Model file for the job. Use its own axes, mm. Give positions to 0.01 mm unless a question says otherwise; leave off trailing zeros. Loops run counter-clockwise (first coordinate to the right, second up) from the corner with the lowest first, then second, coordinate; pieces in that order, holes last. Notation, with made-up numbers: M 70.25,83.5 L 119.25,83.5 A18 ccw 119.25,109.5 Z; hole C -11,73.25 d1. An arc over 180 degrees is marked long. Answer in a Markdown table with one row per item.
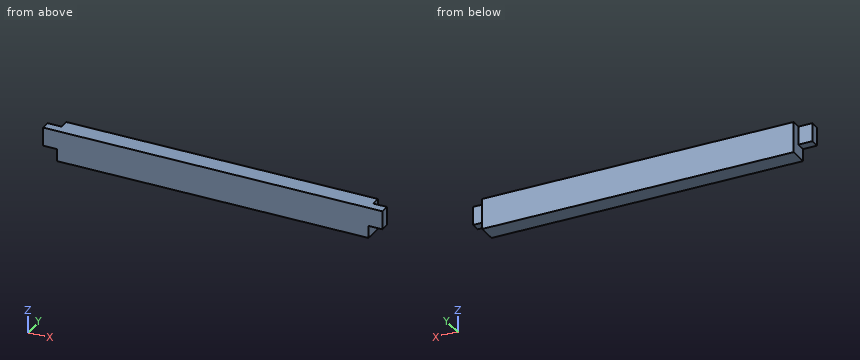
```python
from build123d import *

# Parameters (mm, degrees)
EXTRUDE_1_DEPTH        = 26
EXTRUDE_2_DEPTH        = 19
FILLET_1_R             = 10
SKETCH_1_5_W           = 11
SKETCH_1_5_H           = 340
EXTRUDE_4_DEPTH        = 7
SKETCH_6_W             = 1.9
SKETCH_6_H             = 2
SKETCH_6_W_2           = 6.6
EXTRUDE_5_DEPTH        = 28
SKETCH_6_3_W           = 6.6
SKETCH_6_3_H           = 2
CUT_EXTRUDE_2_DEPTH    = 5
FILLET_2_R             = 20
SKETCH_6_4_W           = 15
SKETCH_6_4_H           = 10
SKETCH_6_4_H_2         = 9
EXTRUDE_6_DEPTH        = 30
SKETCH_6_5_W           = 15
SKETCH_6_5_H           = 9
EXTRUDE_7_DEPTH        = 28
EXTRUDE_8_DEPTH        = 15
FILLET_3_R             = 20
FILLET_3_OF_MIRROR_2_R = 20
FILLET_4_R             = 20
SKETCH_10_W            = 161
SKETCH_10_H            = 20
SKETCH_10_W_2          = 14
EXTRUDE_9_DEPTH        = 7
SKETCH_12_W            = 33
SKETCH_12_H            = 20
CUT_EXTRUDE_3_DEPTH    = 42
SKETCH_11_W            = 19.8
SKETCH_11_H            = 9.8
EXTRUDE_10_DEPTH       = 15


with BuildPart() as part:
    # 스케치1 → 보스-돌출1 (new body)
    with BuildSketch(Plane.XY):
        Polygon((-168, 0), (168, 0), (183, 0), (183, -340), (168, -340), (168, -20), (-168, -20), (-168, -340), (-183, -340), (-183, 0), align=None)
    extrude(amount=EXTRUDE_1_DEPTH)

    # 스케치1<4> → 보스-돌출2 (add)
    with BuildSketch(Plane.XY):
        Polygon((172, 0), (168, 0), (168, -20), (168, -340), (172, -340), align=None)
        Polygon((-168, -20), (-168, 0), (-172, 0), (-172, -340), (-168, -340), align=None)
    extrude(amount=-EXTRUDE_2_DEPTH)

    # 필렛1
    fillet_1_edges = [part.edges().sort_by_distance(p)[0] for p in [
        (170, 0, -19),
        (170, -340, -19),
        (-170, -340, -19),
        (-170, 0, -19),
    ]]
    fillet(fillet_1_edges, radius=FILLET_1_R)

    # 스케치1<5> → 보스-돌출4 (add)
    with BuildSketch(Plane.XY):
        with Locations((177.5, -170)):
            Rectangle(SKETCH_1_5_W, SKETCH_1_5_H)
        with Locations((-177.5, -170)):
            Rectangle(SKETCH_1_5_W, SKETCH_1_5_H)
    extrude(amount=-EXTRUDE_4_DEPTH)

    # 스케치6 → 보스-돌출5 (add)
    with BuildSketch(Plane.XZ.offset(340)):
        with Locations((-182.05, -6)):
            Rectangle(SKETCH_6_W, SKETCH_6_H)
        with Locations((-177.8, -6)):
            Rectangle(SKETCH_6_W_2, SKETCH_6_H)
        Polygon((-174.5, -7), (-172, -7), (-168, -7), (-168, -5), (-174.5, -5), align=None)
    extrude_5 = extrude(amount=EXTRUDE_5_DEPTH)

    # 스케치6<3> → 컷-돌출2 (cut)
    with BuildSketch(Plane.XZ.offset(340)):
        with Locations((-177.8, -6)):
            Rectangle(SKETCH_6_3_W, SKETCH_6_3_H)
    cut_extrude_2 = extrude(amount=CUT_EXTRUDE_2_DEPTH, mode=Mode.SUBTRACT)

    # 필렛2
    # the kernel refuses this fillet: 20 mm, written as the material it adds along each edge
    with BuildSketch(Plane(origin=(-172, -340, -7), x_dir=(0, -1, 0), z_dir=(1, 0, 0))) as fillet_2_piece_1:
        with BuildLine():
            CenterArc((14, 20), FILLET_2_R, 216.869897646, 53.130102354)
            Line((-2, 8), (-3.6, 6.8))
            ThreePointArc((-3.6, 6.8), (-2, 2), (-2, 0))
            Line((-2, 0), (0, -2))
            Line((0, -2), (14, -2))
            Line((14, -2), (14, 0))
        make_face()
    extrude(amount=4)

    # 스케치6<4> → 보스-돌출6 (add)
    with BuildSketch(Plane.XZ.offset(340)):
        with Locations((-175.5, 31)):
            Rectangle(SKETCH_6_4_W, SKETCH_6_4_H)
        with Locations((-175.5, 40.5)):
            Rectangle(SKETCH_6_4_W, SKETCH_6_4_H_2)
    extrude_6 = extrude(amount=-EXTRUDE_6_DEPTH)

    # 스케치6<5> → 보스-돌출7 (add)
    with BuildSketch(Plane.XZ.offset(340)):
        with Locations((-175.5, 40.5)):
            Rectangle(SKETCH_6_5_W, SKETCH_6_5_H)
    extrude_7 = extrude(amount=EXTRUDE_7_DEPTH)

    # 스케치9 → 보스-돌출8 (add)
    with BuildSketch(Plane.ZY.offset(183)):
        Polygon((26, -310), (45, -310), (26, -270), align=None)
    extrude_8 = extrude(amount=-EXTRUDE_8_DEPTH)

    # 필렛3
    fillet_3_edges = [part.edges().sort_by_distance(p)[0] for p in [
        (-175.5, -310, 45),
        (-175.5, -270, 26),
    ]]
    fillet(fillet_3_edges, radius=FILLET_3_R)

    # 대칭 복사2: 보스-돌출5, 컷-돌출2, 보스-돌출6, 보스-돌출7, 보스-돌출8 across plane
    add(extrude_5.mirror(Plane(origin=(0, 0, 0), x_dir=(0, 0, 1), z_dir=(1, 0, 0))))
    add(cut_extrude_2.mirror(Plane(origin=(0, 0, 0), x_dir=(0, 0, 1), z_dir=(1, 0, 0))), mode=Mode.SUBTRACT)
    add(extrude_6.mirror(Plane(origin=(0, 0, 0), x_dir=(0, 0, 1), z_dir=(1, 0, 0))))
    add(extrude_7.mirror(Plane(origin=(0, 0, 0), x_dir=(0, 0, 1), z_dir=(1, 0, 0))))
    add(extrude_8.mirror(Plane(origin=(0, 0, 0), x_dir=(0, 0, 1), z_dir=(1, 0, 0))))

    # 필렛3 of 대칭 복사2
    fillet_3_of_mirror_2_edges = [part.edges().sort_by_distance(p)[0] for p in [
        (175.5, -310, 45),
        (175.5, -270, 26),
    ]]
    fillet(fillet_3_of_mirror_2_edges, radius=FILLET_3_OF_MIRROR_2_R)

    # 필렛4
    # the kernel refuses this fillet: 20 mm, written as the material it adds along each edge
    with BuildSketch(Plane(origin=(172, -340, -7), x_dir=(0, -1, 0), z_dir=(-1, 0, 0))) as fillet_4_piece_1:
        with BuildLine():
            CenterArc((14, -20), FILLET_4_R, 90, 53.130102354)
            Line((-2, -8), (-3.6, -6.8))
            ThreePointArc((-3.6, -6.8), (-2, -2), (-2, 0))
            Line((-2, 0), (0, 2))
            Line((0, 2), (14, 2))
            Line((14, 2), (14, 0))
        make_face()
    extrude(amount=4)

    # 스케치10 → 보스-돌출9 (add)
    with BuildSketch(Plane(origin=(0, 0, 0), x_dir=(-1, 0, 0), z_dir=(0, 0, -1))):
        with Locations((87.5, -10)):
            Rectangle(SKETCH_10_W, SKETCH_10_H)
        with Locations((-87.5, -10)):
            Rectangle(SKETCH_10_W, SKETCH_10_H)
        with Locations((0, -10)):
            Rectangle(SKETCH_10_W_2, SKETCH_10_H)
    extrude(amount=EXTRUDE_9_DEPTH)

    # 스케치12 → 컷-돌출3 (cut)
    with BuildSketch(Plane(origin=(-168, 0, 0), x_dir=(0, 0, -1), z_dir=(1, 0, 0))):
        with BuildLine():
            ThreePointArc((-43.065550087, -305.927473868), (-44.510394688, -310.110371974), (-45, -314.508610159))
            Line((-45, -314.508610159), (-45, -368))
            Line((-45, -368), (-36, -368))
            Line((-36, -368), (-36, -340))
            Line((-36, -340), (5, -340))
            Line((5, -340), (5, -368))
            Line((5, -368), (7, -368))
            Line((7, -368), (7, -354))
            Line((7, -354), (7, -20))
            Line((7, -20), (-26, -20))
            Line((-26, -20), (-26, -265.491389841))
            ThreePointArc((-26, -265.491389841), (-26.489605312, -269.889628026), (-27.934449913, -274.072526132))
            Line((-27.934449913, -274.072526132), (-43.065550087, -305.927473868))
        make_face()
        with Locations((-9.5, -10)):
            Rectangle(SKETCH_12_W, SKETCH_12_H)
        with BuildLine():
            Line((7, 0), (7, -20))
            Line((7, -20), (7, -354))
            ThreePointArc((7, -354), (9.11145618, -345.05572809), (15, -338))
            ThreePointArc((15, -338), (17.94427191, -334.472135955), (19, -330))
            Line((19, -330), (19, -10))
            ThreePointArc((19, -10), (16.071067812, -2.928932188), (9, 0))
            Line((9, 0), (7, 0))
        make_face()
    cut_extrude_3 = extrude(amount=-CUT_EXTRUDE_3_DEPTH, mode=Mode.SUBTRACT)

    # 대칭 복사3: 컷-돌출3 across plane
    add(cut_extrude_3.mirror(Plane(origin=(0, 0, 0), x_dir=(0, 0, 1), z_dir=(1, 0, 0))), mode=Mode.SUBTRACT)

    # 스케치11 → 보스-돌출10 (add)
    with BuildSketch(Plane(origin=(183, 0, 0), x_dir=(0, 0, -1), z_dir=(1, 0, 0))):
        with Locations((-16.1, -15.1)):
            Rectangle(SKETCH_11_W, SKETCH_11_H)
    extrude_10 = extrude(amount=-EXTRUDE_10_DEPTH)

    # 대칭 복사4: 보스-돌출10 across plane
    add(extrude_10.mirror(Plane(origin=(0, 0, 0), x_dir=(0, 0, 1), z_dir=(1, 0, 0))))


solid = part.part
```
(1) Saw through at A-A, the plane z = 10.5. Give the cut face in (x, y), and give its area (3 significant figures).
Established:
| item | result |
|---|---|
| outline | M -183,-20 L 183,-20 L 183,-10.2 L 168,-10.2 L 168,0 L -168,0 L -168,-10.2 L -183,-10.2 Z |
| area | 7,010 mm2 |
(2) Flat gauge pins, fed straight in: P1, Ø7.5, axis at x = 174.5, z = 13, coming from the +Y side; P2, Ø6, axis at y = -2, z = 12, coming from the +X side; P3, Ø3, axis at x = -175.5, y = -17.5, coming from the -Z side. Where does each tip first touch, or does it go through?
Established:
| item | result |
|---|---|
| P1 | stops at y = -10.2 |
| P2 | stops at x = 168 |
| P3 | stops at z = 6.2 |
(3) Saw through at B-B, the plane y = -16. Give the cut face in (x, z), and give its area (3 significant figures).
Established:
| item | result |
|---|---|
| outline | M -183,6.2 L -168,6.2 L -168,-7 L 168,-7 L 168,6.2 L 183,6.2 L 183,26 L -183,26 Z |
| area | 11,700 mm2 |
(4) Wall check: L1, parallel to X at y = -2.75, z = 9.5. Give the ranges that are in metal, low to high.
Established:
| item | result |
|---|---|
| L1 | x = -168 to 168 |
